```python
from build123d import *

# Parameters (mm, degrees)
BOSS_EXTRUDE1_DEPTH = 3.175


with BuildPart() as part:
    # Sketch1 → Boss-Extrude1 (new body)
    with BuildSketch(Plane.XY):
        with BuildLine():
            Line((-50.8, 12.7), (-50.8, 0))
            Line((-50.8, 0), (-44.45, 0))
            Line((-44.45, 0), (-44.45, 3.175))
            Line((-44.45, 3.175), (-39.0144, 3.175))
            Line((-39.0144, 3.175), (-39.0144, 6.858))
            Line((-39.0144, 6.858), (-40.6654, 6.858))
            Line((-40.6654, 6.858), (-40.6654, 9.652))
            Line((-40.6654, 9.652), (-34.3154, 9.652))
            Line((-34.3154, 9.652), (-34.3154, 6.858))
            Line((-34.3154, 6.858), (-35.9664, 6.858))
            Line((-35.9664, 6.858), (-35.9664, 3.175))
            Line((-35.9664, 3.175), (-29.0322, 3.175))
            Line((-29.0322, 3.175), (-29.0322, 6.858))
            Line((-29.0322, 6.858), (-30.6832, 6.858))
            Line((-30.6832, 6.858), (-30.6832, 9.652))
            Line((-30.6832, 9.652), (-24.3332, 9.652))
            Line((-24.3332, 9.652), (-24.3332, 6.858))
            Line((-24.3332, 6.858), (-25.9842, 6.858))
            Line((-25.9842, 6.858), (-25.9842, 3.175))
            Line((-25.9842, 3.175), (-19.05, 3.175))
            Line((-19.05, 3.175), (-19.05, 0))
            Line((-19.05, 0), (0, 0))
            add(Edge.make_bspline(
                [(0, 0), (43.75699028, 0), (90.568040393, -44.45), (127, -44.45)],
                knots=[0, 0, 0, 0, 1, 1, 1, 1], degree=3))
            Line((127, -44.45), (127, -38.354))
            Line((127, -38.354), (123.317, -38.354))
            Line((123.317, -38.354), (123.317, -40.005))
            Line((123.317, -40.005), (120.523, -40.005))
            Line((120.523, -40.005), (120.523, -33.655))
            Line((120.523, -33.655), (123.317, -33.655))
            Line((123.317, -33.655), (123.317, -35.306))
            Line((123.317, -35.306), (127, -35.306))
            Line((127, -35.306), (127, -33.0835))
            Line((127, -33.0835), (130.175, -33.0835))
            Line((130.175, -33.0835), (130.175, -29.9085))
            Line((130.175, -29.9085), (127, -29.9085))
            Line((127, -29.9085), (127, -27.686))
            Line((127, -27.686), (123.317, -27.686))
            Line((123.317, -27.686), (123.317, -29.337))
            Line((123.317, -29.337), (120.523, -29.337))
            Line((120.523, -29.337), (120.523, -22.987))
            Line((120.523, -22.987), (123.317, -22.987))
            Line((123.317, -22.987), (123.317, -24.638))
            Line((123.317, -24.638), (127, -24.638))
            Line((127, -24.638), (127, -19.05))
            add(Edge.make_bspline(
                [(0, 19.05), (43.75699028, 19.05), (89.987535232, -19.05), (127, -19.05)],
                knots=[0, 0, 0, 0, 1, 1, 1, 1], degree=3))
            Line((0, 19.05), (-44.45, 19.05))
            ThreePointArc((-44.45, 19.05), (-48.940128061, 17.190128061), (-50.8, 12.7))
        make_face()
    extrude(amount=BOSS_EXTRUDE1_DEPTH)


solid = part.part
```
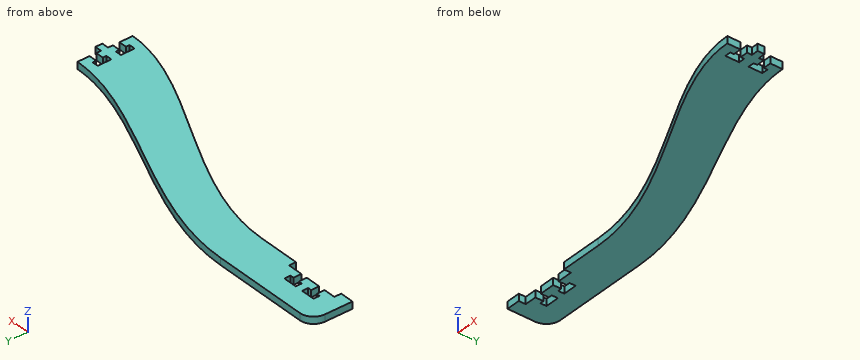
Here's how the part is built. I have some questions about the finished solid (model axes, mm). Give positions to 0.01 mm unless a question says otherwise; leave off trailing zeros. Write each loop counter-clockwise with the first axis right and the second up, starting at its lowest first coordinate (ties: lowest second). Pieces come first, ordered by that corner, then holes. Notation, with made-up numbers: M -31,14.5 L 16,14.5 A24 ccw 16,50.5 Z; hole C -5,29 d6. An arc over 180 degrees is marked long. Put each result on its own line as item: value. Start each with the question number.
Item 1: I need wall thicknesses on L1, parallel to Y at x = -38.5, z = 1.5; L2, parallel to X at y = 5, z = 2.9; L3, parallel to Y at x = 110.5, z = 1.8. Which ranges of each line are inside material? Lowest first, please. Write a range as from..to.
Item 2: Will these pins go through, and if not, where does the flat tip stop? pin 1 (1.6 mm diameter, centred on y = -40, z = 2.5, fed in from +X); pin 2 (1 mm diameter, centred on x = 124.5, z = 2, fed in from +Y); pin 3 (1.5 mm diameter, centred on x = 23.5, z = 1, fed in from +Y).
Item 3: If we section it at A-A, the plane x = -11: Write out the boundary of the cut face in (y, z) (3 decimals), then the cut area to 3 significant figures.
Values:
1. L1: 9.65..19.05
1. L2: -50.8..-39.01, -35.97..-29.03, -25.98..54.47
1. L3: -41.91..-16.91
2. pin 1: x = 127
2. pin 2: y = -18.97
2. pin 3: y = 16.05
3. outline: M 0,0 L 19.05,0 L 19.05,3.175 L 0,3.175 Z
3. area: 60.5 mm²
